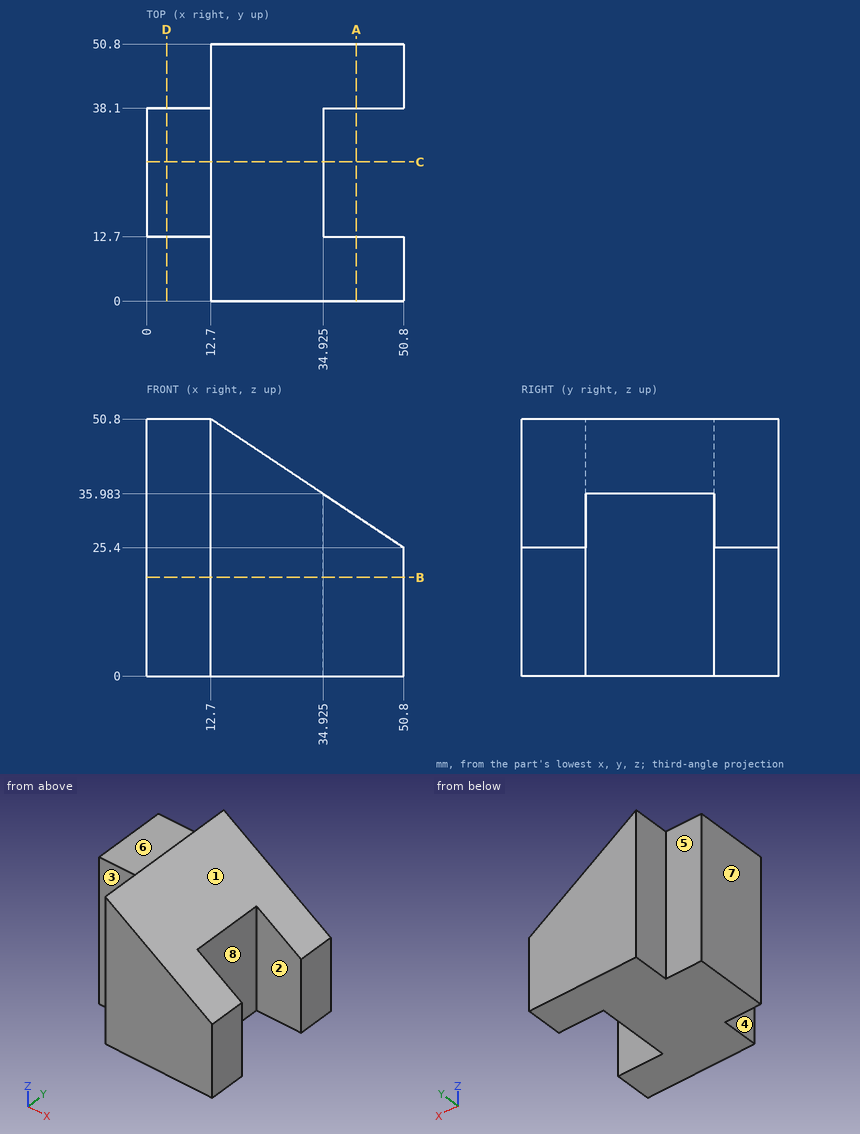
Job drawing, mm, ordinate dimensions from the low corner. One solid piece. A direction names the side the tool comes from. Coordinates: 2 decimals unless noted, no trailing zeros. Write each loop counter-clockwise with the first axis right and the second up, starting at its lowest first coordinate (ties: lowest second). Pieces come first, ordered by that corner, then holes. Notation, with made-up numbers: (17, 51.25) - (36, 51.25) arc R21 ccw to (36, 75.25) - close; hole circle Ø9 at (4.5, 10.25). An arc over 180 degrees is marked (long way). Use a Markdown table: item, result. Add a question column.
Item 1: Band-saw the part on D-D, the plane x = 4. Give the cut face in (y, z).
Item 2: Band-saw the part on C-C, the plane y = 27.5. Give the cut face in (x, z) (1 decimal), and give its area (3 significant figures).
Item 3: Mould opens along Y. For the marked faces 1, 2 and 3 say: pulls with the +Y half, pulls with the -Y half, needs draft (parallel to the pull), parting line crosses it, or undercut.
Item 4: Band-saw the part on B-B, the plane z = 19.5. Give the cut face in (x, y) (1 decimal).
Item 5: 3-axis set-ups, long thin cutter, end or side, ignore diameter. For the marked faces 4, 5, 6, 7 and 8: which of +Z, -Z, +X, -X, +Y, -Y reach the whole face in a straight line?
Item 6: Drill centre lines: L1, parallel to Y at x = 41, z = 18; L2, parallel to X at y = 16.5, z = 26 (1 decimal); L3, parallel to Y at x = 7, z = 17. Where is each one in solid material? Low to high. Write a range as from..to.
Item 7: Flat gauge pins, fed straight in: pin 1 (14 mm diameter, centred on x = 3.5, z = 20, fed in from -Y); pin 2 (6 mm diameter, centred on x = 30.5, y = 10, fed in from +Z); pin 3 (6.5 mm diameter, centred on x = 4.5, z = 36, fed in from +Y). Where does each tip first touch, or does it go through?
Item 8: Band-saw the part on A-A, the plane x = 41.5. Give the cut face in (y, z).
Numbers:
| question | item | result |
|---|---|---|
| 1 | outline | (12.7, 0) - (38.1, 0) - (38.1, 50.8) - (12.7, 50.8) - close |
| 2 | outline | (0, 0) - (34.9, 0) - (34.9, 36) - (12.7, 50.8) - (0, 50.8) - close |
| 2 | area | 1,610 mm2 |
| 3 | face 1 | needs draft |
| 3 | face 2 | undercut |
| 3 | face 3 | pulls with the -Y half |
| 4 | outline | (0, 12.7) - (12.7, 12.7) - (12.7, 0) - (50.8, 0) - (50.8, 12.7) - (34.9, 12.7) - (34.9, 38.1) - (50.8, 38.1) - (50.8, 50.8) - (12.7, 50.8) - (12.7, 38.1) - (0, 38.1) - close |
| 5 | face 4 | +Z, -Z, -X, -Y |
| 5 | face 5 | +Z, -Z, -X, +Y |
| 5 | face 6 | +Z, +X, -X, +Y, -Y |
| 5 | face 7 | +Z, -Z, -X, +Y, -Y |
| 5 | face 8 | +Z, -Z, +X |
| 6 | L1 | 0..12.7, 38.1..50.8 |
| 6 | L2 | 0..34.9 |
| 6 | L3 | 12.7..38.1 |
| 7 | pin 1 | y = 12.7 |
| 7 | pin 2 | z = 40.93 |
| 7 | pin 3 | y = 38.1 |
| 8 | outline | (0, 0) - (12.7, 0) - (12.7, 31.6) - (0, 31.6) - close; (38.1, 0) - (50.8, 0) - (50.8, 31.6) - (38.1, 31.6) - close |
